from build123d import *

# Parameters (mm, degrees)
F1_DEPTH = 26
F3_DEPTH = 25
F5_D     = 10


with BuildPart() as f1:
    # F0 (on Top) → F1 (new body)
    with BuildSketch(Plane.XY):
        with BuildLine():
            Line((-38.8, 5), (-38.8, 0))
            Line((-38.8, 0), (0, 0))
            Line((0, 0), (17.632412, 29.941532))
            Line((17.632412, 29.941532), (34.95292, 19.941532))
            Line((34.95292, 19.941532), (39.95292, 28.601786))
            Line((39.95292, 28.601786), (13.972158, 43.601786))
            Line((13.972158, 43.601786), (-3.984466, 12.5))
            ThreePointArc((-3.984466, 12.5), (-5.814593, 10.669873), (-8.314593, 10))
            Line((-8.314593, 10), (-33.8, 10))
            ThreePointArc((-33.8, 10), (-37.335534, 8.535534), (-38.8, 5))
        make_face()
    extrude(amount=F1_DEPTH)

    # F2 (on face) → F3 (cut)
    with BuildSketch(Plane(origin=(0, 10, 0), x_dir=(-1, 0, 0), z_dir=(0, 1, 0))):
        with BuildLine():
            ThreePointArc((27.3, 11.5), (28.36066, 11.93934), (28.8, 13))
            ThreePointArc((28.8, 13), (28.36066, 14.06066), (27.3, 14.5))
            ThreePointArc((27.3, 14.5), (25.8, 13), (27.3, 11.5))
        make_face()
        with BuildLine():
            ThreePointArc((15.8, 13), (15.36066, 14.06066), (14.3, 14.5))
            ThreePointArc((14.3, 14.5), (12.8, 13), (14.3, 11.5))
            ThreePointArc((14.3, 11.5), (15.36066, 11.93934), (15.8, 13))
        make_face()
        with BuildLine():
            ThreePointArc((27.3, 11.5), (25.8, 13), (27.3, 14.5))
            Line((27.3, 14.5), (14.3, 14.5))
            ThreePointArc((14.3, 14.5), (15.36066, 14.06066), (15.8, 13))
            ThreePointArc((15.8, 13), (15.36066, 11.93934), (14.3, 11.5))
            Line((14.3, 11.5), (27.3, 11.5))
        make_face()
    extrude(amount=-F3_DEPTH, mode=Mode.SUBTRACT)

    # F5 (through all)
    with Locations(Plane.XZ):
        with Locations((26.483979, 13)):
            Hole(F5_D / 2)


solid = f1.part
For this review, take the finished solid that the model builds, in its own axes (mm). A direction names the side the tool comes from. Coordinates: 2 decimals unless noted, no trailing zeros. Order: outer loops, then holes, each group sorted by start corner. A loop starts at its lowest first (then second) coordinate and runs counter-clockwise, first axis right, second up. Notation, with made-up numbers: (73.25, -9) - (79.25, -9) arc R18 cw to (79.25, 1) - close; hole circle Ø9 at (82, 41). An arc over 180 degrees is marked (long way). Answer as CSV lines item,"result". Start each with the question number.
1) To check wall thickness, follow line 1 along Z through (x, y) = (-26.5, 3); line 2 along X through (y, z) = (5, 12.75); line 3 along Y through (x, z) = (-19.5, 17.5). State the ranges of each line that lie inside material, in increasing order. Write a range as [from, to].
2) Draft analysis for pull direction Z (two halves, no side actions). For faces 6 (the flat face through (0, 17, 0)), 7 (the flat face through (0, 17, 26)), 8 (the cylindrical face through (-12.8, 5.1, 13)), state which applies: +Z half, -Z half, draft (parallel to the pull), parting line (faces both ways), or undercut.
3) Machinability: for faces 1 (the flat face through (8.69, 14.76, 12.82)), 2 (the flat face through (-38.8, 3, 13)), 3 (the flat face through (-21, 10, 10)), 4 (the flat face through (-20, 0, 10)), 5 (the flat face through (-21, 5, 14.5)), which of the approach directions +Z, -Z, +X, -X, +Y, -Y give a long, thin tool a straight path to every point of the face, cutting with its end or side? Answer none if there is none.
4) Insertion check: P1, Ø6, axis at y = 17.5, z = 6.5, coming from the -X side; P2, Ø12, axis at y = 26.5, z = 5.5, coming from the -X side; P3, Ø12, axis at x = 12, y = 6, coming from the +Z side; P4, Ø1.5, axis at y = 33, z = 11, coming from the +X side. Each pin has a flat end and moves straight along its axis. Give the tip position at first contact, or say it passes through.
5) Add section A-A (z = 21.25). State the section outline as (x, y) points, then the cut area to 3 significant figures.
6) Add section B-B (y = 24.5). State the section outline as (x, z) points, then the cut area to 3 significant figures.
7) Add section D-D (y = 8). State the section outline as (x, z) points.
8) Add section C-C (z = 10.75). State the section outline as (x, y) points, then the cut area to 3 significant figures.
Result:
1,line 1,"[0, 11.5], [14.5, 26]"
1,line 2,"[-38.8, -28.78], [-12.82, 2.94]"
1,line 3,"[0, 10]"
2,face 6,"-Z half"
2,face 7,"+Z half"
2,face 8,"undercut"
3,face 1,"+Z, -Z, -Y"
3,face 2,"+Z, -Z, -X, +Y, -Y"
3,face 3,"+Z, -Z, -X, +Y"
3,face 4,"+Z, -Z, +X, -X, -Y"
3,face 5,"+Y, -Y"
4,P1,"x = -2.83"
4,P2,"x = 0.63"
4,P3,"through"
4,P4,"x = 33.63"
5,outline,"(-38.8, 0) - (0, 0) - (17.63, 29.94) - (34.95, 19.94) - (39.95, 28.6) - (13.97, 43.6) - (-3.98, 12.5) arc R5 cw to (-8.31, 10) - (-33.8, 10) arc R5 ccw to (-38.8, 5) - close"
5,area,"970 mm^2"
6,outline,"(2.94, 0) - (14.43, 0) - (14.43, 26) - (2.94, 26) - close; (27.06, 0) - (37.58, 0) - (37.58, 26) - (27.06, 26) - (27.06, 17.97) arc R5 cw to (27.06, 8.03) - close"
6,area,"539 mm^2"
7,outline,"(-37.8, 0) - (4.71, 0) - (4.71, 26) - (-37.8, 26) - close; hole (-28.8, 13) arc R1.5 ccw to (-27.3, 11.5) - (-14.3, 11.5) arc R1.5 ccw to (-14.3, 14.5) - (-27.3, 14.5) arc R1.5 ccw to start"
8,outline,"(-38.8, 0) - (0, 0) - (17.63, 29.94) - (22.02, 27.41) - (22.02, 38.96) - (13.97, 43.6) - (-3.98, 12.5) arc R5 cw to (-8.31, 10) - (-33.8, 10) arc R5 ccw to (-38.8, 5) - close; (30.95, 22.25) - (34.95, 19.94) - (39.95, 28.6) - (30.95, 33.8) - close"
8,area,"867 mm^2"
